Geometry check sheet. Reference: the model listing, model coordinates, mm. Give positions to 0.01 mm unless a question says otherwise; leave off trailing zeros.
from build123d import *

# Parameters (mm, degrees)
F0_W     = 88.9
F0_H     = 1715.224484
F0_R     = 12.7
F1_DEPTH = 19.05
F3_DEPTH = 88.901


with BuildPart() as f1:
    # F0 (on Front) → F1 (new body)
    with BuildSketch(Plane.XZ):
        with Locations((-1388.109314, -537.817911)):
            Rectangle(F0_W, F0_H)
        with Locations((-1388.109314, -1248.586403)):
            Circle(F0_R, mode=Mode.SUBTRACT)
        with Locations((-1388.109314, -1172.386403)):
            Circle(F0_R, mode=Mode.SUBTRACT)
        with Locations((-1388.109314, -1096.186403)):
            Circle(F0_R, mode=Mode.SUBTRACT)
        with Locations((-1388.109314, -812.023903)):
            Circle(F0_R, mode=Mode.SUBTRACT)
        with Locations((-1388.109314, -735.823903)):
            Circle(F0_R, mode=Mode.SUBTRACT)
        with Locations((-1388.109314, -659.623903)):
            Circle(F0_R, mode=Mode.SUBTRACT)
        with Locations((-1388.109314, -365.936403)):
            Circle(F0_R, mode=Mode.SUBTRACT)
        with Locations((-1388.109314, -289.736403)):
            Circle(F0_R, mode=Mode.SUBTRACT)
        with Locations((-1388.109314, -213.536403)):
            Circle(F0_R, mode=Mode.SUBTRACT)
        with Locations((-1388.109314, -6.367653)):
            Circle(F0_R, mode=Mode.SUBTRACT)
        with Locations((-1388.109314, 69.832347)):
            Circle(F0_R, mode=Mode.SUBTRACT)
        with Locations((-1388.109314, 146.032347)):
            Circle(F0_R, mode=Mode.SUBTRACT)
    extrude(amount=F1_DEPTH)

    # F2 (on face) → F3 (cut, through all)
    with BuildSketch(Plane(origin=(-1432.559314, 0, 0), x_dir=(0, -1, 0), z_dir=(-1, 0, 0))):
        Polygon((19.05, 319.794331), (0, 319.794331), (19.05, 278.785859), align=None)
    extrude(amount=-F3_DEPTH, mode=Mode.SUBTRACT)


solid = f1.part
Item 1: Sectioned sample at A-A (y = -14.75). Give the number of separate pieces and of enclosed holes in the cut face, and give its area (3 significant figures).
Reported:
separate pieces: 1
enclosed holes: 12
area: 144,000 mm2
Item 2: Gauge pin test, flat ends, axial feed: pin 1 (10 mm diameter, centred on x = -1370, y = -10.5, fed in from +Z); pin 2 (20.5 mm diameter, centred on x = -1388.11, z = -289.74, fed in from +Y); pin 3 (2 mm diameter, centred on x = -1366.5, y = -14, fed in from +Z); pin 4 (3 mm diameter, centred on x = -1403.5, y = -11.5, fed in from +Z). Record the tip position at first contact, or that the pin passes through.
Reported:
pin 1: stops at z = 307.95
pin 2: passes through
pin 3: stops at z = 291.81
pin 4: stops at z = 298.27
Item 3: Scan lines: L1, parallel to X at y = -9.5, z = 140.5; L2, parallel to X at y = -8.25, z = -656; L3, parallel to Z at x = -1372, y = -9.5. Record each from-to range of solid material in increasing order.
Reported:
L1: x = -1432.56 to -1399.54, -1376.68 to -1343.66
L2: x = -1432.56 to -1400.28, -1375.94 to -1343.66
L3: z = -1395.43 to 299.34
